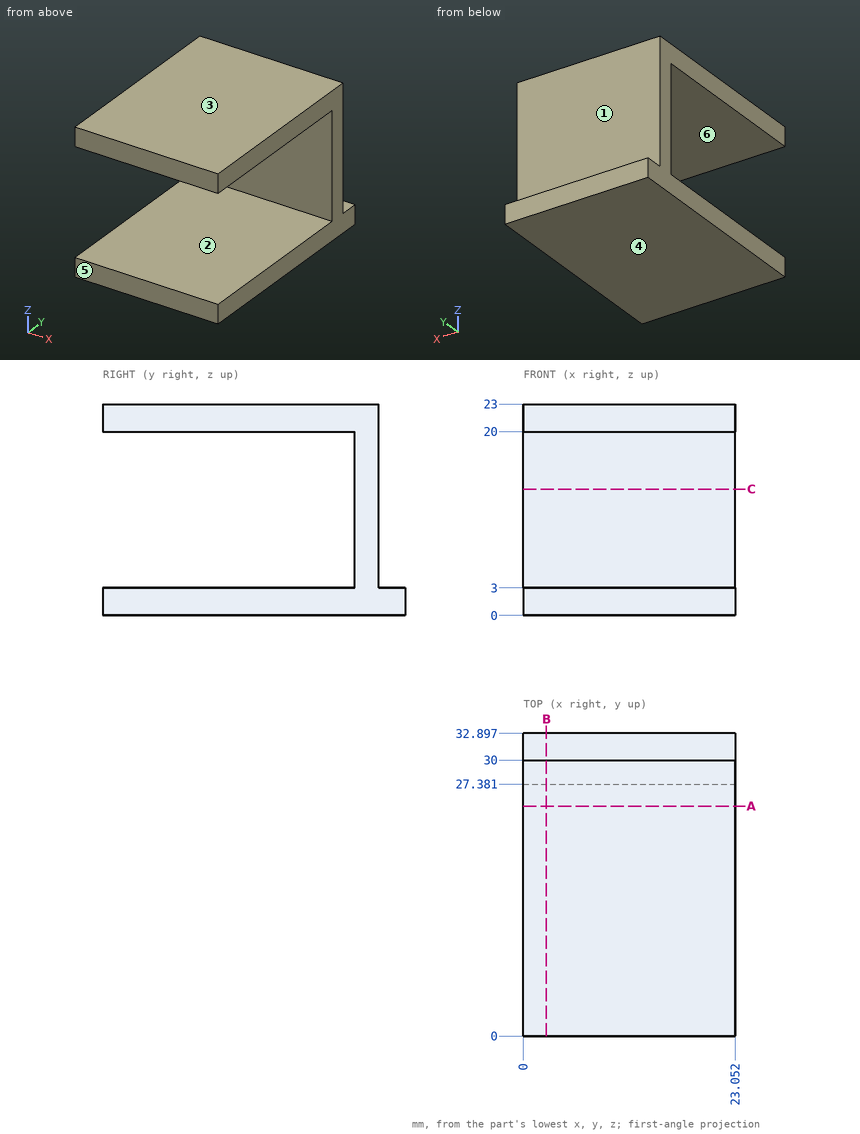
Study the drawing (mm; zero at the part's minimum x, y, z) and answer. A direction names the side the tool comes from. Coordinates: 2 decimals unless noted, no trailing zeros. Loops run counter-clockwise (first coordinate to the right, second up) from the corner with the lowest first, then second, coordinate; pieces in that order, holes last. Notation, with made-up numbers: M -11.75,79.25 L -0.75,79.25 A15 ccw -0.75,93.25 Z; hole C 50.5,48 d7. An arc over 180 degrees is marked long. Answer as a JSON object with one key per item and string values. Group by question number.
Item 1: Which of the six approach directions +Z, -Z, +X, -X, +Y, -Y give full straight-line access (tool end or side, diameter ignored) to the marked faces 1, 2 and 3?
Item 2: Consider L1, parallel to Z at x = 14.25, y = 9; L2, parallel to Y at x = 7.5, z = 10; L3, parallel to Y at x = 6.5, z = 20.75. Determine where each line is inside the solid, lowest interval first.
Item 3: Determine the mould class of the marked faces 4, 5 and 6 for opening direction Z: +Z half, -Z half, draft (parallel to the pull), parting line (faces both ways), or undercut.
Item 4: Section C-C (z = 13.75) is taken. Write down the section's boundary in (x, y).
Item 5: Section A-A (y = 25) is taken. Write down the section's boundary in (x, z), and give its area (3 significant figures).
Item 6: Section B-B (x = 2.5) is taken. Write down the section's boundary in (y, z), and give its area (3 significant figures).
Item 7: Each of these flat-tipped pins is pushed along its axis until it touches: P1, Ø10, axis at x = 10, z = 16, coming from the +Y side; P2, Ø5, axis at x = 10, z = 14.5, coming from the -Y side; P3, Ø5, axis at y = 21.5, z = 6, coming from the +X side; P4, Ø2.5, axis at x = 12, y = 32, coming from the +Z side. Where does it stop, or does it pass through?
Solved:
{
 "1": {"face 1": "+Z, +X, -X, +Y", "face 2": "+X, -X, -Y", "face 3": "+Z, +X, -X, +Y, -Y"},
 "2": {"L1": "z = 0 to 3, 20 to 23", "L2": "y = 27.38 to 30", "L3": "y = 0 to 30"},
 "3": {"face 4": "-Z half", "face 5": "draft", "face 6": "undercut"},
 "4": {"outline": "M 0,27.38 L 23.05,27.38 L 23.05,30 L 0,30 Z"},
 "5": {"outline": "M 0,0 L 23.05,0 L 23.05,3 L 0,3 Z; M 0,20 L 23.05,20 L 23.05,23 L 0,23 Z", "area": "138 mm2"},
 "6": {"outline": "M 0,0 L 32.9,0 L 32.9,3 L 30,3 L 30,23 L 0,23 L 0,20 L 27.38,20 L 27.38,3 L 0,3 Z", "area": "233 mm2"},
 "7": {"P1": "stops at y = 30", "P2": "stops at y = 27.38", "P3": "passes through", "P4": "stops at z = 3"}
}
